Autodesk Inventor part; units mm, degrees
ref_plane "YZ Plane" through (0, 0, 0) normal (1, 0, 0) x (0, 1, 0)
ref_plane "XZ Plane" through (0, 0, 0) normal (0, 1, 0) x (-1, 0, 0)
ref_plane "XY Plane" through (0, 0, 0) normal (0, 0, 1) x (1, 0, 0)
sketch "Sketch1" plane through (0, 0, 0) normal (0, 0, 1) x (1, 0, 0)
  line L0 (-64.749, 104.525) -> (-139.8022, 4.926) construction
  line L1 (0, 104.525) -> (-64.749, 104.525) construction
  line L2 (-139.8022, 4.926) -> (-218.9225, -165.525) construction
  line L3 (0, -219.535) -> (0, 158.535) construction
  line L4 (64.749, 104.525) -> (139.8022, 4.926) construction
  line L5 (0, 104.525) -> (64.749, 104.525) construction
  line L6 (139.8022, 4.926) -> (218.9225, -165.525) construction
  line L7 (-218.9225, -165.525) -> (0, -165.525) construction
  line L8 (218.9225, -165.525) -> (0, -165.525) construction
  line L9 (-62.7547, 100.525) -> (-136.3525, 2.8574) construction
  line L10 (-136.3525, 2.8574) -> (-212.6558, -161.525)
  line L11 (-212.6558, -161.525) -> (0, -161.525)
  line L12 (0, -161.525) -> (212.6558, -161.525)
  line L13 (212.6558, -161.525) -> (136.3525, 2.8574)
  line L14 (136.3525, 2.8574) -> (62.7547, 100.525) construction
  line L15 (62.7547, 100.525) -> (0, 100.525) construction
  line L16 (0, 100.525) -> (-62.7547, 100.525) construction
  line L17 (-136.3525, 2.8574) -> (-131.8312, 8.8574)
  line L18 (-131.8312, 8.8574) -> (0, 8.8574)
  line L19 (136.3525, 2.8574) -> (131.8312, 8.8574)
  line L20 (131.8312, 8.8574) -> (0, 8.8574)
  point P0 (0, 0)
  dimension "d0" = 4
  dimension "d34" = 6
extrude "Plate1" add sketch "Sketch1" along normal blind 3.048
fillet "Fillet1" radius 8 6 edges at (-212.6558, -161.525, 1.524) (212.6558, -161.525, 1.524) (-131.8312, 8.8574, 1.524) (-136.3525, 2.8574, 1.524) (131.8312, 8.8574, 1.524) (136.3525, 2.8574, 1.524)
sketch "Sketch3" plane through (0, 0, 3.048) normal (0, 0, 1) x (1, 0, 0)
  arc A0 (200.1225, -161.525) -> (207.3789, -150.1567) centre (200.1225, -153.525) ccw construction
  line L0 (136.7095, 2.0883) -> (207.3789, -150.1567) construction
  line L1 (-207.3789, -150.1567) -> (-136.7095, 2.0883) construction
  arc A1 (-207.3789, -150.1567) -> (-200.1225, -161.525) centre (-200.1225, -153.525) ccw construction
  line L2 (200.1225, -161.525) -> (-200.1225, -161.525) construction
  line L3 (-59.7632, 94.525) -> (59.7632, 94.525) construction
  line L4 (59.7632, 94.525) -> (131.178, -0.2457) construction
  line L5 (131.178, -0.2457) -> (203.2558, -155.525) construction
  line L6 (203.2558, -155.525) -> (-203.2558, -155.525) construction
  line L7 (-203.2558, -155.525) -> (-131.178, -0.2457) construction
  line L8 (-131.178, -0.2457) -> (-59.7632, 94.525) construction
  circle A2 centre (-59.7632, 94.525) radius 3
  circle A3 centre (59.7632, 94.525) radius 3
  circle A4 centre (-131.178, -0.2457) radius 3
  circle A5 centre (131.178, -0.2457) radius 3
  circle A6 centre (-200.1225, -153.525) radius 3
  line L9 (0, -215.7211) -> (0, 149.7327) construction
  circle A7 centre (200.1225, -153.525) radius 3
  arc A8 (136.7095, 2.0883) -> (135.8422, 3.5345) centre (129.4531, -1.28) ccw
  line L10 (134.2316, 5.6719) -> (135.8422, 3.5345)
  arc A9 (134.2316, 5.6719) -> (127.8425, 8.8574) centre (127.8425, 0.8574) ccw
  line L11 (-127.8425, 8.8574) -> (127.8425, 8.8574)
  arc A10 (-127.8425, 8.8574) -> (-134.2316, 5.6719) centre (-127.8425, 0.8574) ccw
  line L12 (-135.8422, 3.5345) -> (-134.2316, 5.6719)
  arc A11 (-135.8422, 3.5345) -> (-136.7095, 2.0883) centre (-129.4531, -1.28) ccw
  point P0 (0, 0)
  dimension "d4" = 6
extrude "Cut1" cut sketch "Sketch3" against normal blind 3.048
sketch "Sketch5" plane through (0, 0, 3.048) normal (0, 0, 1) x (1, 0, 0)
  circle A0 centre (-131.178, -0.2457) radius 3 construction
  circle A1 centre (131.178, -0.2457) radius 3 construction
  circle A2 centre (-200.1225, -153.525) radius 3 construction
  circle A3 centre (200.1225, -153.525) radius 3 construction
  arc A4 (136.7095, 2.0883) -> (135.8422, 3.5345) centre (129.4531, -1.28) ccw construction
  line L0 (134.2316, 5.6719) -> (135.8422, 3.5345) construction
  arc A5 (134.2316, 5.6719) -> (127.8425, 8.8574) centre (127.8425, 0.8574) ccw construction
  line L1 (-127.8425, 8.8574) -> (127.8425, 8.8574) construction
  arc A6 (-127.8425, 8.8574) -> (-134.2316, 5.6719) centre (-127.8425, 0.8574) ccw construction
  line L2 (-135.8422, 3.5345) -> (-134.2316, 5.6719) construction
  arc A7 (-135.8422, 3.5345) -> (-136.7095, 2.0883) centre (-129.4531, -1.28) ccw construction
  line L3 (-207.3789, -150.1567) -> (-136.7095, 2.0883) construction
  arc A8 (-207.3789, -150.1567) -> (-200.1225, -161.525) centre (-200.1225, -153.525) ccw construction
  line L4 (200.1225, -161.525) -> (-200.1225, -161.525) construction
  arc A9 (200.1225, -161.525) -> (207.3789, -150.1567) centre (200.1225, -153.525) ccw construction
  line L5 (136.7095, 2.0883) -> (207.3789, -150.1567) construction
  line L6 (0, -198.138) -> (0, 44.2342) construction
  line L7 (-100, 8.8574) -> (-100, -161.525) construction
  line L8 (-207.3789, -150.1567) -> (-136.7095, 2.0883)
  line L9 (200.1225, -161.525) -> (-200.1225, -161.525)
  line L10 (-15, -7.1426) -> (15, -7.1426) construction
  line L11 (15, -7.1426) -> (0, -33.1234) construction
  line L12 (0, -33.1234) -> (-15, -7.1426) construction
  circle A10 centre (-15, -7.1426) radius 3
  circle A11 centre (15, -7.1426) radius 3
  circle A12 centre (0, -33.1234) radius 3
  circle A13 centre (-100, -38.1039) radius 3
  circle A14 centre (-100, -142.6039) radius 3
  circle A15 centre (100, -38.1039) radius 3
  circle A16 centre (100, -142.6039) radius 3
  line L13 (0, -54.1039) -> (-72.5, -126.6039)
  line L14 (-72.5, -126.6039) -> (72.5, -126.6039)
  line L15 (72.5, -126.6039) -> (0, -54.1039)
  line L16 (-84.1532, -115.1039) -> (-23.1532, -54.1039)
  line L17 (-23.1532, -54.1039) -> (-145.1532, -54.1039)
  line L18 (-145.1532, -54.1039) -> (-84.1532, -115.1039)
  line L19 (-152.4933, -69.9169) -> (-95.8064, -126.6039)
  line L20 (-95.8064, -126.6039) -> (-178.8064, -126.6039)
  line L21 (-178.8064, -126.6039) -> (-152.4933, -69.9169)
  line L22 (-145.1532, -54.1039) -> (-152.4933, -69.9169) construction
  line L23 (-23.1532, -54.1039) -> (0, -54.1039) construction
  line L24 (-95.8064, -126.6039) -> (-72.5, -126.6039) construction
  line L25 (-84.1532, -115.1039) -> (-84.1532, -126.6039) construction
  line L26 (84.1532, -115.1039) -> (23.1532, -54.1039)
  line L27 (23.1532, -54.1039) -> (145.1532, -54.1039)
  line L28 (145.1532, -54.1039) -> (84.1532, -115.1039)
  line L29 (152.4933, -69.9169) -> (95.8064, -126.6039)
  line L30 (95.8064, -126.6039) -> (178.8064, -126.6039)
  line L31 (178.8064, -126.6039) -> (152.4933, -69.9169)
  point P0 (0, 0)
  point P1 (0, -7.1426)
  dimension "d38" = 60
  dimension "d39" = 30
  dimension "d40" = 16
  dimension "d41" = 6
  dimension "d54" = 100
  dimension "d57" = 45
  dimension "d58" = 16
  dimension "d59" = 16
  dimension "d60" = 145
  dimension "d61" = 122
  dimension "d62" = 83
  dimension "d63" = 16
extrude "Cut3" cut sketch "Sketch5" against normal blind 3.048 contours A10 | A11 | A12 | L15 L14 L13 | L18 L17 L16 | L19 L20 L21 | L26 L27 L28 | L31 L30 L29
fillet "Fillet3" radius 8 15 edges at (72.5, -126.6039, 1.524) (0, -54.1039, 1.524) (-72.5, -126.6039, 1.524) (-178.8064, -126.6039, 1.524) (-152.4933, -69.9169, 1.524) (-95.8064, -126.6039, 1.524) (178.8064, -126.6039, 1.524) (95.8064, -126.6039, 1.524) (152.4933, -69.9169, 1.524) (145.1532, -54.1039, 1.524) (84.1532, -115.1039, 1.524) (23.1532, -54.1039, 1.524) (-84.1532, -115.1039, 1.524) (-145.1532, -54.1039, 1.524) (-23.1532, -54.1039, 1.524)
equation "\"d4\" = d3"
equation "\"d5\" = Thickness"
equation "\"d1\" = Thickness"
equation "\"BendRadius\" = Thickness"
equation "\"BendReliefWidth\" = Thickness"
equation "\"BendReliefDepth\" = 0.5 * Thickness"
equation "\"CornerReliefSize\" = 4 * Thickness"
equation "\"MinimumRemnant\" = 2 * Thickness"
equation "\"TransitionRadius\" = BendRadius"
equation "\"JacobiRadiusSize\" = BendRadius"
equation "\"GapSize\" = Thickness"
properties part number "ChestFront"
Design review of the part built by this model. Coordinates are the model's own, in mm. A direction names the side the tool comes from. Give positions to 0.01 mm unless a question says otherwise; leave off trailing zeros. Order: outer loops, then holes, each group sorted by start corner. A loop starts at its lowest first (then second) coordinate and runs counter-clockwise, first axis right, second up. Notation, with made-up numbers: (26, 59.25) - (64, 59.25) arc R36 cw to (64, 95.25) - close; hole circle Ø6 at (20.25, 1.25). An arc over 180 degrees is marked (long way). Use a Markdown table: item, result. Add a question column.
(1) Wall thickness on probe 1 along X at (y, z) = (-121.5, 0.2); probe 2 along X at (y, z) = (-115, 1.55); probe 3 along Y at (x, z) = (15, 1.8) (3 decimals): over which ranges is each line inside the solid? List them lowest first. Write a range as [from, to].
(2) Add section C-C on z = 0.85. Give the number of separate pieces and of enclosed holes in the cut face, then the cut area to 3 significant figures.
(3) Add section B-B on y = -89. Give the boundary of the cut face in (x, z), then the cut area to 3 significant figures.
(4) Clearance check with flat-ended pins moving along their axes: P1, Ø7, axis at x = -15, y = -7.14, coming from the +Z side; P2, Ø0.9, axis at x = 131, z = 2, coming from the +Y side. State where each tip first meets the part, or that it passes through.
(5) Add section D-D on y = -24.5. Give the boundary of the cut face in (x, z), then the cut area to 3 significant figures.
(6) Add section A-A on x = -96. Give the boundary of the cut face in (y, z) (3 decimals).
(7) Mouldability with a two-part tool opening along Y and no side actions: class faces 3 (the face through (-3, -56, 0)), 4 (the face through (-171.55, -72.97, 1.5)), 5 (the face through (-172.955, -123.002, 1.503)) as +Y half, -Y half, draft (parallel to the pull), parting line (faces both ways), or undercut.
(8) Machinability: for faces 1 (the face through (-31.878, -85.982, 1.545)), 2 (the face through (-3, -56, 3.048)), which of the approach directions +Z, -Z, +X, -X, +Y, -Y give a long, thin tool a straight path to every point of the face, cutting with its end or side? Answer none if there is none.
Report:
| question | item | result |
|---|---|---|
| 1 | probe 1 | x = [-194.08, -173.73], [-107.66, -60.64], [60.64, 107.66], [173.73, 194.08] |
| 1 | probe 2 | x = [-191.06, -173.42], [-107.98, -60.33], [60.33, 107.98], [173.42, 191.06] |
| 1 | probe 3 | y = [-161.525, -126.604], [-69.104, -10.143], [-4.143, 8.857] |
| 2 | separate pieces | 1 |
| 2 | enclosed holes | 12 |
| 2 | area | 42,100 mm² |
| 3 | outline | (-178.99, 0) - (-161.35, 0) - (-161.35, 3.05) - (-178.99, 3.05) - close; (-133.41, 0) - (-110.26, 0) - (-110.26, 3.05) - (-133.41, 3.05) - close; (-58.05, 0) - (-34.9, 0) - (-34.9, 3.05) - (-58.05, 3.05) - close; (34.9, 0) - (58.05, 0) - (58.05, 3.05) - (34.9, 3.05) - close; (110.26, 0) - (133.41, 0) - (133.41, 3.05) - (110.26, 3.05) - close; (161.35, 0) - (178.99, 0) - (178.99, 3.05) - (161.35, 3.05) - close |
| 3 | area | 390 mm² |
| 4 | P1 | stops at z = 3.05 |
| 4 | P2 | stops at y = 8.39 |
| 5 | outline | (-149.05, 0) - (149.05, 0) - (149.05, 3.05) - (-149.05, 3.05) - close |
| 5 | area | 909 mm² |
| 6 | outline | (-161.525, 0) - (-103.257, 0) - (-103.257, 3.048) - (-161.525, 3.048) - close; (-54.104, 0) - (8.857, 0) - (8.857, 3.048) - (-54.104, 3.048) - close |
| 7 | face 3 | draft |
| 7 | face 4 | +Y half |
| 7 | face 5 | undercut |
| 8 | face 1 | +Z, -Z |
| 8 | face 2 | +Z, +X, -X, +Y, -Y |
